Job drawing, mm, ordinate dimensions from the low corner. One solid piece. A direction names the side the tool comes from. Round coordinates to 2 decimals unless told otherwise and drop trailing zeros. Write each loop counter-clockwise with the first axis right and the second up, starting at its lowest first coordinate (ties: lowest second). Pieces come first, ordered by that corner, then holes. Notation, with made-up numbers: M 69,83 L 117,83 A12 cw 117,104 Z; hole C 75.5,74 d6. An arc over 180 degrees is marked long. Answer as a JSON object with one key per item and string values. Group by question number.
1. Drop flat-ended pins along their axis: pin 1 (1 mm diameter, centred on y = 3.5, z = 4, fed in from +X); pin 2 (1.8 mm diameter, centred on x = 3, y = 8, fed in from -Z). Give the stop position or say it passes through.
2. Drill centre lines: line 1 (Y direction, x = 8, z = 4.05); line 2 (X direction, y = 7.25, z = 1.55) (1 decimal); line 3 (X direction, y = 5, z = 0.65). Where is each one in solid material? Low to high. Write a range as from..to.
3. Which spindle directions (+Z, -Z, +X, -X, +Y, -Y) get a long thin tool onto all of the face, cutting with end or side? Do the marked faces 5 and 6. Say none if no direction does.
4. Band-saw the part on B-B, the plane z = 4.65. Write the cut outline in (x, y).
5. Band-saw the part on A-A, the plane z = 1.25. Write the cut outline in (x, y), plus the area to 3 significant figures.
6. Two-plate mould, pull along X, no slides. Class the marked faces 1, 2, 3 and 4: +X half, -X half, draft (parallel to the pull), parting line (faces both ways), or undercut.
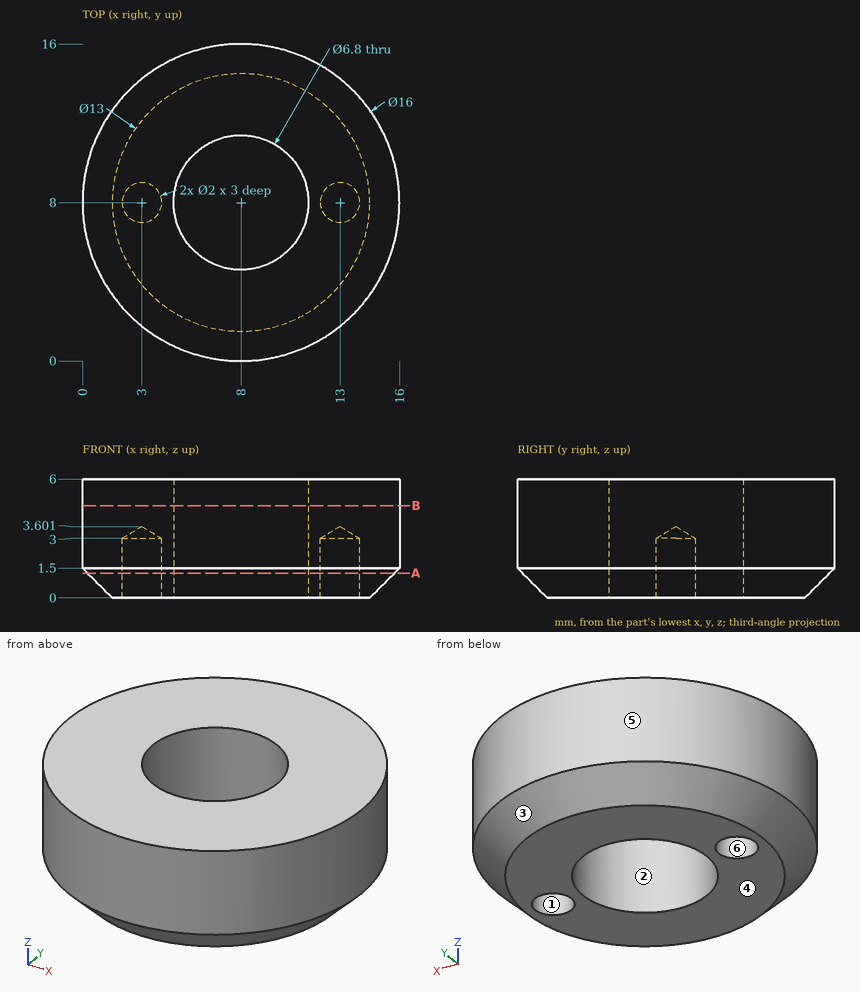
Worked answers:
{
 "1": {"pin 1": "stops at x = 14.93", "pin 2": "stops at z = 3.06"},
 "2": {"line 1": "y = 0..4.6, 11.4..16", "line 2": "x = 0..2.3, 3.7..4.7, 11.3..12.3, 13.7..16", "line 3": "x = 1.51..6.4, 9.6..14.49"},
 "3": {"face 5": "+Z, -Z", "face 6": "-Z"},
 "4": {"outline": "C 8,8 d16; hole C 8,8 d6.8"},
 "5": {"outline": "C 8,8 d15.5; hole C 3,8 d2; hole C 8,8 d6.8; hole C 13,8 d2", "area": "146 mm^2"},
 "6": {"face 1": "undercut", "face 2": "undercut", "face 3": "parting line", "face 4": "draft"}
}
